Design review of the part built by this model. Coordinates are the model's own, in mm. A direction names the side the tool comes from. Round coordinates to 2 decimals unless told otherwise and drop trailing zeros. Loops run counter-clockwise (first coordinate to the right, second up) from the corner with the lowest first, then second, coordinate; pieces in that order, holes last. Notation, with made-up numbers: M -34,74 L -2,74 A21 ccw -2,98 Z; hole C 44,54 d10. An arc over 180 degrees is marked long. Use a Markdown table: item, result.
from build123d import *

# Parameters (mm, degrees)
F1_DEPTH = 2400


with BuildPart() as f1:
    # F0 (on Top) → F1 (new body)
    with BuildSketch(Plane.XY):
        with BuildLine():
            Line((-4, 0), (0, 0))
            Line((0, 0), (0, 108.361391))
            ThreePointArc((0, 108.361391), (0.16233, 109.74761), (0.640534, 111.058821))
            Line((0.640534, 111.058821), (16.564311, 142.69743))
            ThreePointArc((16.564311, 142.69743), (18.776125, 145.108061), (21.923777, 146))
            Line((21.923777, 146), (41, 146))
            ThreePointArc((41, 146), (45.242641, 144.242641), (47, 140))
            Line((47, 140), (47, 125))
            Line((47, 125), (51, 125))
            Line((51, 125), (51, 144))
            ThreePointArc((51, 144), (49.242641, 148.242641), (45, 150))
            Line((45, 150), (19.458927, 150))
            ThreePointArc((19.458927, 150), (16.311275, 149.108061), (14.099461, 146.69743))
            Line((14.099461, 146.69743), (-3.359466, 112.008665))
            ThreePointArc((-3.359466, 112.008665), (-3.83767, 110.697454), (-4, 109.311235))
            Line((-4, 109.311235), (-4, 0))
        make_face()
    extrude(amount=F1_DEPTH)


solid = f1.part
1. Machinability: for faces 1 (the face through (-1, 98, 2400)), 2 (the face through (0, 53, 1183)), which of the approach directions +Z, -Z, +X, -X, +Y, -Y give a long, thin tool a straight path to every point of the face, cutting with its end or side? Answer none if there is none.
Check values:
| item | result |
|---|---|
| face 1 | +Z, +X, -X, +Y, -Y |
| face 2 | +Z, -Z, +X, -Y |
2. Take a section at B-B on y = 34. Give the boundary of the cut face in (x, z), and give its area (3 significant figures).
Check values:
| item | result |
|---|---|
| outline | M -4,0 L 0,0 L 0,2400 L -4,2400 Z |
| area | 9,600 mm² |
3. Insertion check: pin 1 (10 mm diameter, centred on x = 22.5, z = 1275, fed in from -Y); pin 2 (5.5 mm diameter, centred on x = 32, z = 1794, fed in from -Y); pin 3 (2 mm diameter, centred on x = 48.5, z = 1107.5, fed in from -Y). Each pin has a flat end and moves straight along its axis. Give the tip position at first contact, or say it passes through.
Check values:
| item | result |
|---|---|
| pin 1 | stops at y = 144.05 |
| pin 2 | stops at y = 146 |
| pin 3 | stops at y = 125 |
4. Take a section at A-A on z = 2194. Give the boundary of the cut face in (x, y).
Check values:
| item | result |
|---|---|
| outline | M -4,0 L 0,0 L 0,108.36 A6 cw 0.64,111.06 L 16.56,142.7 A6 cw 21.92,146 L 41,146 A6 cw 47,140 L 47,125 L 51,125 L 51,144 A6 ccw 45,150 L 19.46,150 A6 ccw 14.1,146.7 L -3.36,112.01 A6 ccw -4,109.31 Z |
5. Wall thickness on line 1 along Y through (x, z) = (36.5, 1250.5); line 2 along Y through (x, z) = (43, 255); line 3 along X through (y, z) = (43, 636.5): over which ranges is each line inside the solid? List them lowest first. Write a range as from..to.
Check values:
| item | result |
|---|---|
| line 1 | y = 146..150 |
| line 2 | y = 145.66..150 |
| line 3 | x = -4..0 |
